```python
from build123d import *

# Parameters (mm, degrees)
SKETCH_1_R      = 10
SKETCH_1_R_2    = 1.6
EXTRUDE_1_DEPTH = 2
SKETCH_2_R      = 4.5
SKETCH_2_R_2    = 2.75
EXTRUDE_2_DEPTH = 2.5


with BuildPart() as part:
    # 草图1 → 凸台-拉伸1 (new body)
    with BuildSketch(Plane.XY):
        Circle(SKETCH_1_R)
        with Locations((0, 7)):
            Circle(SKETCH_1_R_2, mode=Mode.SUBTRACT)
        with Locations((7, 0)):
            Circle(SKETCH_1_R_2, mode=Mode.SUBTRACT)
        with Locations((0, -7)):
            Circle(SKETCH_1_R_2, mode=Mode.SUBTRACT)
        with Locations((-7, 0)):
            Circle(SKETCH_1_R_2, mode=Mode.SUBTRACT)
    extrude(amount=EXTRUDE_1_DEPTH)

    # 草图2 → 凸台-拉伸2 (add)
    with BuildSketch(Plane(origin=(0, 0, 0), x_dir=(-1, 0, 0), z_dir=(0, 0, -1))):
        Circle(SKETCH_2_R)
        Circle(SKETCH_2_R_2, mode=Mode.SUBTRACT)
    extrude(amount=EXTRUDE_2_DEPTH)


solid = part.part
```
Design review of the part built by this model. Coordinates are the model's own, in mm. A direction names the side the tool comes from. Give positions to 0.01 mm unless a question says otherwise; leave off trailing zeros. Write each loop counter-clockwise with the first axis right and the second up, starting at its lowest first coordinate (ties: lowest second). Pieces come first, ordered by that corner, then holes. Notation, with made-up numbers: (28.5, 29.5) -> (58.5, 29.5) arc R11 ccw to (58.5, 40.5) -> close; hole circle Ø11 at (10, 79.25). An arc over 180 degrees is marked (long way). Answer in a Markdown table with one row per item.
(1) To check wall thickness, follow probe 1 along Y at (x, z) = (0, 1.3); probe 2 along Y at (x, z) = (1, 1.45); probe 3 along Y at (x, z) = (0, -1.2). State the ranges of each line that lie inside material, in increasing order.
Results:
| item | result |
|---|---|
| probe 1 | -10 to -8.6, -5.4 to 5.4, 8.6 to 10 |
| probe 2 | -9.95 to -8.25, -5.75 to 5.75, 8.25 to 9.95 |
| probe 3 | -4.5 to -2.75, 2.75 to 4.5 |
(2) Clearance check with flat-ended pins moving along their axes: pin 1 (4 mm diameter, centred on x = -4.5, y = -0.5, fed in from -Z); pin 2 (4 mm diameter, centred on x = 7, y = 0, fed in from -Z); pin 3 (2.5 mm diameter, centred on x = 0, y = -7, fed in from -Z). State where each tip first meets the part, or that it passes through.
Results:
| item | result |
|---|---|
| pin 1 | z = -2.5 |
| pin 2 | z = 0 |
| pin 3 | through |
(3) For faces 1 (the cylindrical face through (-0.35, -8.56, 0.99)), 2 (the cylindrical face through (0.596, -2.685, -1.232)), list the 3-axis set-ups (+Z, -Z, +X, -X, +Y, -Y) from which the entire face can be reached by the end or side of a thin tool; tool diameter is ignored.
Results:
| item | result |
|---|---|
| face 1 | +Z, -Z |
| face 2 | -Z |
(4) Consider section C-C (z = 1.4). State the section outline as (x, y) points, then the cut area to 3 significant figures.
Results:
| item | result |
|---|---|
| outline | circle Ø20 at (0, 0); hole circle Ø3.2 at (-7, 0); hole circle Ø3.2 at (0, -7); hole circle Ø3.2 at (0, 7); hole circle Ø3.2 at (7, 0) |
| area | 282 mm2 |
(5) Mouldability with a two-part tool opening along Y and no side actions: class faces 3 (the flat face through (4.3, -2.1, 0)), 4 (the cylindrical face through (-8.6, 0.07, 0.99)), 5 (the cylindrical face through (5.4, 0.07, 0.99)), 6 (the cylindrical face through (-2.17, -9.76, 0.99)) as +Y half, -Y half, draft (parallel to the pull), parting line (faces both ways), or undercut.
Results:
| item | result |
|---|---|
| face 3 | draft |
| face 4 | undercut |
| face 5 | undercut |
| face 6 | parting line |
(6) Consider section A-A (y = 5.75). State the section outline as (x, z) points, then the cut area to 3 significant figures.
Results:
| item | result |
|---|---|
| outline | (-8.18, 0) -> (-1, 0) -> (-1, 2) -> (-8.18, 2) -> close; (1, 0) -> (8.18, 0) -> (8.18, 2) -> (1, 2) -> close |
| area | 28.7 mm2 |
(7) Consider section B-B (x = -7.5). State the section outline as (y, z) points.
Results:
| item | result |
|---|---|
| outline | (-6.61, 0) -> (-1.52, 0) -> (-1.52, 2) -> (-6.61, 2) -> close; (1.52, 0) -> (6.61, 0) -> (6.61, 2) -> (1.52, 2) -> close |
(8) Consider section D-D (x = -0.25). State the section outline as (y, z) points, then the cut area to 3 significant figures.
Results:
| item | result |
|---|---|
| outline | (-10, 0) -> (-8.58, 0) -> (-8.58, 2) -> (-10, 2) -> close; (-5.42, 0) -> (-4.49, 0) -> (-4.49, -2.5) -> (-2.74, -2.5) -> (-2.74, 0) -> (2.74, 0) -> (2.74, -2.5) -> (4.49, -2.5) -> (4.49, 0) -> (5.42, 0) -> (5.42, 2) -> (-5.42, 2) -> close; (8.58, 0) -> (10, 0) -> (10, 2) -> (8.58, 2) -> close |
| area | 36.1 mm2 |
